```python
from build123d import *

# Parameters (mm, degrees)
F1_FACE_R   = 17
F1_FACE_R_2 = 16
F3_DEPTH    = 1.2
F4_T1_DEPTH = 1.2


# Not quite as in the source:
# - a fillet or chamfer that OpenCascade refuses, or shapes differently, is made with other operations: its cross-section is extruded or revolved along the edge and cut away or added


with BuildPart() as f1:
    # F0 (on Front) → F1 (revolve)
    with BuildSketch(Plane.XZ):
        with BuildLine():
            Line((-5, -6.2), (-5, -7))
            Line((-5, -7), (-1.8672954017, -7))
            ThreePointArc((-1.8672954017, -7), (-1.2120936603, -6.755453955), (-0.877345908, -6.1414213562))
            Line((-0.877345908, -6.1414213562), (0, 0))
            Line((0, 0), (-1, 0))
            Line((-1, 0), (-1.8643923288, -5.3592324388))
            ThreePointArc((-1.8643923288, -5.3592324388), (-2.2032633542, -5.9613253046), (-2.8516334496, -6.2))
            Line((-2.8516334496, -6.2), (-5, -6.2))
        make_face()
    revolve(axis=Axis((16, 0, -3.4995676855), (0, 0, -1)))

    # F1_face (on face) + F2 (on Top) → F3 (join)
    with BuildSketch(Plane(origin=(16, 0, 0), x_dir=(1, 0, 0), z_dir=(0, 0, 1))):
        Circle(F1_FACE_R)
        Circle(F1_FACE_R_2, mode=Mode.SUBTRACT)
    with BuildSketch(Plane.XY):
        with BuildLine():
            Line((3.7233340059, 0.6), (0.0112539579, 0.6))
            ThreePointArc((0.0112539579, 0.6), (0, 0), (0.0112539579, -0.6))
            Line((0.0112539579, -0.6), (3.7233340059, -0.6))
            ThreePointArc((3.7233340059, -0.6), (7.3688969309, -8.8359634953), (15.6048604261, -12.4815264202))
            Line((15.6048604261, -12.4815264202), (15.6048604261, -15.9951200282))
            ThreePointArc((15.6048604261, -15.9951200282), (16.2050046444, -15.9986866053), (16.8048604261, -15.9797434177))
            Line((16.8048604261, -15.9797434177), (16.8048604261, -12.4815264202))
            ThreePointArc((16.8048604261, -12.4815264202), (25.0408239214, -8.8359634953), (28.6863868464, -0.6))
            Line((28.6863868464, -0.6), (31.9887460421, -0.6))
            ThreePointArc((31.9887460421, -0.6), (31.9971862631, -0.3000527668), (32, 0))
            ThreePointArc((32, 0), (31.9971862631, 0.3000527668), (31.9887460421, 0.6))
            Line((31.9887460421, 0.6), (28.6863868464, 0.6))
            ThreePointArc((28.6863868464, 0.6), (25.0408239214, 8.8359634953), (16.8048604261, 12.4815264202))
            Line((16.8048604261, 12.4815264202), (16.8048604261, 15.9797434177))
            ThreePointArc((16.8048604261, 15.9797434177), (16.2050046444, 15.9986866053), (15.6048604261, 15.9951200282))
            Line((15.6048604261, 15.9951200282), (15.6048604261, 12.4815264202))
            ThreePointArc((15.6048604261, 12.4815264202), (7.3688969309, 8.8359634953), (3.7233340059, 0.6))
        make_face()
        with BuildLine():
            ThreePointArc((15.6048604261, -11.6414250608), (7.9622037717, -8.2426566544), (4.5634353654, -0.6))
            Line((4.5634353654, -0.6), (9.6268322864, -0.6))
            ThreePointArc((9.6268322864, -0.6), (11.5341830552, -4.6706773709), (15.6048604261, -6.5780281397))
            Line((15.6048604261, -6.5780281397), (15.6048604261, -11.6414250608))
        make_face(mode=Mode.SUBTRACT)
        with BuildLine():
            ThreePointArc((15.6048604261, -5.8326828273), (12.0587665437, -4.1460938824), (10.3721775989, -0.6))
            Line((10.3721775989, -0.6), (14.6048604261, -0.6))
            ThreePointArc((14.6048604261, -0.6), (15.3119672073, -0.8928932188), (15.6048604261, -1.6))
            Line((15.6048604261, -1.6), (15.6048604261, -5.8326828273))
        make_face(mode=Mode.SUBTRACT)
        with BuildLine():
            ThreePointArc((16.8048604261, -6.5780281397), (20.875537797, -4.6706773709), (22.7828885658, -0.6))
            Line((22.7828885658, -0.6), (27.8462854869, -0.6))
            ThreePointArc((27.8462854869, -0.6), (24.4475170805, -8.2426566544), (16.8048604261, -11.6414250608))
            Line((16.8048604261, -11.6414250608), (16.8048604261, -6.5780281397))
        make_face(mode=Mode.SUBTRACT)
        with BuildLine():
            ThreePointArc((22.0375432534, -0.6), (20.3509543085, -4.1460938824), (16.8048604261, -5.8326828273))
            Line((16.8048604261, -5.8326828273), (16.8048604261, -1.6))
            ThreePointArc((16.8048604261, -1.6), (17.0977536449, -0.8928932188), (17.8048604261, -0.6))
            Line((17.8048604261, -0.6), (22.0375432534, -0.6))
        make_face(mode=Mode.SUBTRACT)
        with BuildLine():
            ThreePointArc((10.3721775989, 0.6), (12.0587665437, 4.1460938824), (15.6048604261, 5.8326828273))
            Line((15.6048604261, 5.8326828273), (15.6048604261, 1.6))
            ThreePointArc((15.6048604261, 1.6), (15.3119672073, 0.8928932188), (14.6048604261, 0.6))
            Line((14.6048604261, 0.6), (10.3721775989, 0.6))
        make_face(mode=Mode.SUBTRACT)
        with BuildLine():
            ThreePointArc((4.5634353654, 0.6), (7.9622037717, 8.2426566544), (15.6048604261, 11.6414250608))
            Line((15.6048604261, 11.6414250608), (15.6048604261, 6.5780281397))
            ThreePointArc((15.6048604261, 6.5780281397), (11.5341830552, 4.6706773709), (9.6268322864, 0.6))
            Line((9.6268322864, 0.6), (4.5634353654, 0.6))
        make_face(mode=Mode.SUBTRACT)
        with BuildLine():
            Line((16.8048604261, 1.6), (16.8048604261, 5.8326828273))
            ThreePointArc((16.8048604261, 5.8326828273), (20.3509543085, 4.1460938824), (22.0375432534, 0.6))
            Line((22.0375432534, 0.6), (17.8048604261, 0.6))
            ThreePointArc((17.8048604261, 0.6), (17.0977536449, 0.8928932188), (16.8048604261, 1.6))
        make_face(mode=Mode.SUBTRACT)
        with BuildLine():
            Line((16.8048604261, 6.5780281397), (16.8048604261, 11.6414250608))
            ThreePointArc((16.8048604261, 11.6414250608), (24.4475170805, 8.2426566544), (27.8462854869, 0.6))
            Line((27.8462854869, 0.6), (22.7828885658, 0.6))
            ThreePointArc((22.7828885658, 0.6), (20.875537797, 4.6706773709), (16.8048604261, 6.5780281397))
        make_face(mode=Mode.SUBTRACT)
    extrude(amount=F3_DEPTH)

    # F4: fillet of radius 1 on 8 edges, made by hand

    # F4_s2 → F4_t1 (join)
    with BuildSketch(Plane.XY):
        with BuildLine():
            ThreePointArc((14.5118511212, 15.9306438324), (15.2782810581, 15.6742381227), (15.6048604261, 14.9349785929))
            Line((15.6048604261, 14.9349785929), (15.6048604261, 15.9951200282))
            ThreePointArc((15.6048604261, 15.9951200282), (15.0578040841, 15.9722342475), (14.5118511212, 15.9306438324))
        make_face()
        with BuildLine():
            ThreePointArc((17.9251844545, 15.8837547455), (17.1416576021, 15.6394597938), (16.8048604261, 14.8910200739))
            Line((16.8048604261, 14.8910200739), (16.8048604261, 15.9797434177))
            ThreePointArc((16.8048604261, 15.9797434177), (17.3658659227, 15.9415937184), (17.9251844545, 15.8837547455))
        make_face()
        with BuildLine():
            ThreePointArc((31.9087173867, -1.7066666667), (31.6582863368, -0.9316687448), (30.91442255, -0.6))
            Line((30.91442255, -0.6), (31.9887460421, -0.6))
            ThreePointArc((31.9887460421, -0.6), (31.9583276403, -1.1540272632), (31.9087173867, -1.7066666667))
        make_face()
        with BuildLine():
            ThreePointArc((31.9087173867, 1.7066666667), (31.6582863368, 0.9316687448), (30.91442255, 0.6))
            Line((30.91442255, 0.6), (31.9887460421, 0.6))
            ThreePointArc((31.9887460421, 0.6), (31.9583276403, 1.1540272632), (31.9087173867, 1.7066666667))
        make_face()
        with BuildLine():
            ThreePointArc((14.5118511212, -15.9306438324), (15.2782810581, -15.6742381227), (15.6048604261, -14.9349785929))
            Line((15.6048604261, -14.9349785929), (15.6048604261, -15.9951200282))
            ThreePointArc((15.6048604261, -15.9951200282), (15.0578040841, -15.9722342475), (14.5118511212, -15.9306438324))
        make_face()
        with BuildLine():
            ThreePointArc((17.9251844545, -15.8837547455), (17.1416576021, -15.6394597938), (16.8048604261, -14.8910200739))
            Line((16.8048604261, -14.8910200739), (16.8048604261, -15.9797434177))
            ThreePointArc((16.8048604261, -15.9797434177), (17.3658659227, -15.9415937184), (17.9251844545, -15.8837547455))
        make_face()
        with BuildLine():
            ThreePointArc((0.0912826133, 1.7066666667), (0.3417136632, 0.9316687448), (1.08557745, 0.6))
            Line((1.08557745, 0.6), (0.0112539579, 0.6))
            ThreePointArc((0.0112539579, 0.6), (0.0416723597, 1.1540272632), (0.0912826133, 1.7066666667))
        make_face()
        with BuildLine():
            ThreePointArc((0.0912826133, -1.7066666667), (0.3417136632, -0.9316687448), (1.08557745, -0.6))
            Line((1.08557745, -0.6), (0.0112539579, -0.6))
            ThreePointArc((0.0112539579, -0.6), (0.0416723597, -1.1540272632), (0.0912826133, -1.7066666667))
        make_face()
    extrude(amount=F4_T1_DEPTH)


solid = f1.part
```
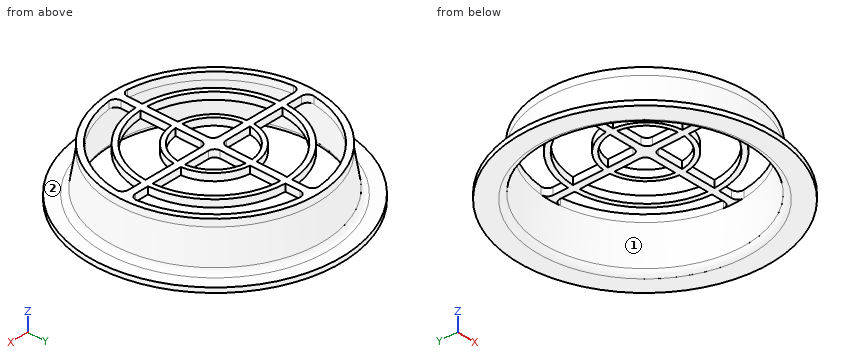
Design review of the part built by this model. Coordinates are the model's own, in mm. Face numbers are marked on the shaded views. A direction names the side the tool comes from. Give positions to 0.01 mm unless a question says otherwise; leave off trailing zeros. Write each loop counter-clockwise with the first axis right and the second up, starting at its lowest first coordinate (ties: lowest second). Pieces come first, ordered by that corner, then holes. Notation, with made-up numbers: (29, 89.5) -> (69, 89.5) arc R24 cw to (69, 102.5) -> close; hole circle Ø1 at (15.5, 58). An arc over 180 degrees is marked (long way). Answer in a Markdown table with one row per item.
(1) Consider section A-A (y = 0). State the section outline as (x, z) points.
Results:
| item | result |
|---|---|
| outline | (-5, -7) -> (-1.87, -7) arc R1 ccw to (-0.88, -6.14) -> (0, 0) -> (32, 0) -> (32.88, -6.14) arc R1 ccw to (33.87, -7) -> (37, -7) -> (37, -6.2) -> (34.85, -6.2) arc R1 cw to (33.86, -5.36) -> (33, 0) -> (33, 1.2) -> (-1, 1.2) -> (-1, 0) -> (-1.86, -5.36) arc R1 cw to (-2.85, -6.2) -> (-5, -6.2) -> close |
(2) For the marked faces 1 and 2, list the 3-axis set-ups (+Z, -Z, +X, -X, +Y, -Y) from which the entire face can be reached by the end or side of a thin tool; tool diameter is ignored.
Results:
| item | result |
|---|---|
| face 1 | -Z |
| face 2 | +Z |
(3) Clearance check with flat-ended pins moving along their axes: pin 1 (3 mm diameter, centred on x = 11, y = -1, fed in from -Z); pin 2 (1.3 mm diameter, centred on x = 13, z = 1, fed in from +Y); pin 3 (1.3 mm diameter, centred on y = 4, z = 0.5, fed in from -X). State where each tip first meets the part, or that it passes through.
Results:
| item | result |
|---|---|
| pin 1 | z = 0 |
| pin 2 | y = 16.84 |
| pin 3 | x = -0.67 |
(4) To check wall thickness, follow probe 1 along Y at (x, z) = (17.5, -4); probe 2 along X at (y, z) = (6, -0.75); probe 3 along Y at (x, z) = (26.5, -4.25). State the ranges of each line that lie inside material, in increasing order.
Results:
| item | result |
|---|---|
| probe 1 | -17.58 to -16.5, 16.5 to 17.58 |
| probe 2 | -0.04 to 1.05, 30.95 to 32.04 |
| probe 3 | -14.23 to -12.87, 12.87 to 14.23 |
(5) Consider section C-C (x = 8.5). Count the separate pieces of the cut face and the enclosed holes in it, then the cut area to 3 significant figures.
Results:
| item | result |
|---|---|
| separate pieces | 5 |
| enclosed holes | 0 |
| area | 28.4 mm2 |
(6) Consider section B-B (z = -3.5). State the section outline as (x, y) points.
Results:
| item | result |
|---|---|
| outline | circle Ø35.13 at (16, 0); hole circle Ø33 at (16, 0) |
